from build123d import *

# Parameters (mm, degrees)
BOSS_EXTRUDE1_DEPTH = 11.4
CUT_EXTRUDE1_DEPTH  = 0.6
CHAMFER1_SIZE       = 0.5
CUT_EXTRUDE2_DEPTH  = 6


with BuildPart() as part:
    # Sketch2 → Boss-Extrude1 (new body)
    with BuildSketch(Plane(origin=(0, 0, 0), x_dir=(1, 0, 0), z_dir=(0, 1, 0))):
        with BuildLine():
            Line((-13.742133053, -2.045066795), (-2.112067201, -2.853361551))
            ThreePointArc((-2.112067201, -2.853361551), (0, -3.55), (2.112067201, -2.853361551))
            Line((2.112067201, -2.853361551), (13.742133053, -2.045066795))
            ThreePointArc((13.742133053, -2.045066795), (15.65, 0), (13.742133053, 2.045066795))
            Line((13.742133053, 2.045066795), (2.112067201, 2.853361551))
            ThreePointArc((2.112067201, 2.853361551), (0, 3.55), (-2.112067201, 2.853361551))
            Line((-2.112067201, 2.853361551), (-13.742133053, 2.045066795))
            ThreePointArc((-13.742133053, 2.045066795), (-15.65, 0), (-13.742133053, -2.045066795))
        make_face()
    extrude(amount=BOSS_EXTRUDE1_DEPTH)

    # Sketch3 → Cut-Extrude1 (cut)
    with BuildSketch(Plane.XZ):
        with BuildLine():
            ThreePointArc((-2.112067201, 2.853361551), (0, -3.55), (2.112067201, 2.853361551))
            ThreePointArc((2.112067201, 2.853361551), (0, 3.55), (-2.112067201, 2.853361551))
        make_face()
    extrude(amount=-CUT_EXTRUDE1_DEPTH, mode=Mode.SUBTRACT)

    # Chamfer1
    chamfer1_edges = [part.edges().sort_by_distance(p)[0] for p in [
        (-3.55, 0, 0),
        (3.55, 0, 0),
    ]]
    chamfer(chamfer1_edges, length=CHAMFER1_SIZE)

    # Shaft Key → Cut-Extrude2 (cut)
    with BuildSketch(Plane(origin=(0, 11.4, 0), x_dir=(1, 0, 0), z_dir=(0, 1, 0))):
        with BuildLine():
            Line((1.6, -1.855397532), (1.6, -5.45))
            Line((1.6, -5.45), (-1.6, -5.45))
            Line((-1.6, -5.45), (-1.6, -1.855397532))
            ThreePointArc((-1.6, -1.855397532), (-2.45, 0), (-1.6, 1.855397532))
            Line((-1.6, 1.855397532), (-1.6, 5.45))
            Line((-1.6, 5.45), (1.6, 5.45))
            Line((1.6, 5.45), (1.6, 1.855397532))
            ThreePointArc((1.6, 1.855397532), (2.45, 0), (1.6, -1.855397532))
        make_face()
    extrude(amount=-CUT_EXTRUDE2_DEPTH, mode=Mode.SUBTRACT)


solid = part.part
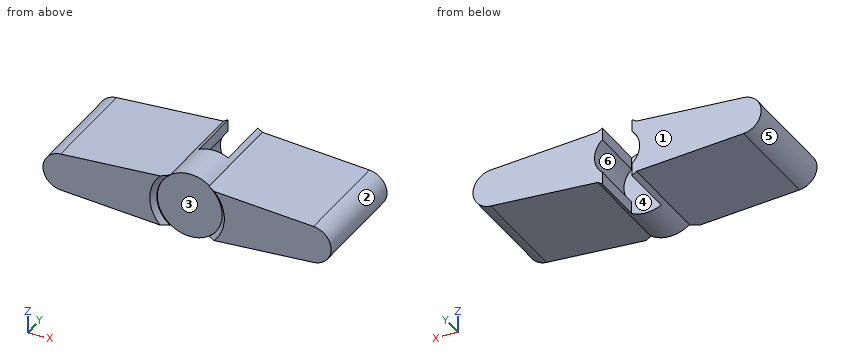
Could you check a few things on this model? Use its own coordinates, in mm. Face numbers are marked on the shaded views. A direction names the side the tool comes from. Give positions to 0.01 mm unless a question says otherwise; leave off trailing zeros. Order: outer loops, then holes, each group sorted by start corner. A loop starts at its lowest first (then second) coordinate and runs counter-clockwise, first axis right, second up.
1. Suppose I cut it at D-D (x = -0.5). Write out the boundary of the cut face in (y, z), plus the area to 3 significant figures.
Answers below:
outline: (0.6, -3.51) - (5.4, -3.51) - (5.4, 3.51) - (0.6, 3.51) - close
area: 33.7 mm2
2. For pin 1 (2.5 mm diameter, centred on x = 0, z = 1, fed in from +Y); pin 2 (1.4 mm diameter, centred on y = 7.5, z = 2.5, fed in from +X); pin 3 (2 mm diameter, centred on x = 1, z = 1.5, fed in from -Y), each with a flat end and sliding along its axis, tell me the tip position at first contact or that it passes through.
Answers below:
pin 1: stops at y = 5.4
pin 2: stops at x = 14.58
pin 3: stops at y = 0.6
3. Suppose I cut it at B-B (y = 3). Write out the boundary of the cut face in (x, z).
Answers below:
outline: (-13.74, -2.05) - (-2.11, -2.85) arc R3.55 ccw to (2.11, -2.85) - (13.74, -2.05) arc R2.05 ccw to (13.74, 2.05) - (2.11, 2.85) arc R3.55 ccw to (-2.11, 2.85) - (-13.74, 2.05) arc R2.05 ccw to start
4. Thinking about a two-plate mould opening in X: for the marked faces 1, 2, 3 and 4, which applies, +X half, -X half, draft (parallel to the pull), parting line (faces both ways), or undercut?
Answers below:
face 1: draft
face 2: +X half
face 3: undercut
face 4: undercut
5. Which directions (+Z, -Z, +X, -X, +Y, -Y) give clear straight access to the entire face, cutting with the end or side of a thin tool? Please do the marked faces 5 and 6.
Answers below:
face 5: -X, +Y, -Y
face 6: +Y
6. Suppose I cut it at C-C (z = 0). Write out the boundary of the cut face in (x, y), plus the area to 3 significant figures.
Answers below:
outline: (-15.65, 0) - (-4.05, 0) - (-3.55, 0.5) - (-3.55, 0.6) - (3.55, 0.6) - (3.55, 0.5) - (4.05, 0) - (15.65, 0) - (15.65, 11.4) - (2.45, 11.4) - (2.45, 5.4) - (-2.45, 5.4) - (-2.45, 11.4) - (-15.65, 11.4) - close
area: 323 mm2
7. I need wall thicknesses on L1, parallel to Y at x = 1.5, z = 1; L2, parallel to X at y = 8.25, z = 0.75; L3, parallel to Z at x = -4, y = 7.25. Which ranges of each line are inside material? Lowest first, please.
Answers below:
L1: y = 0.6 to 5.4
L2: x = -15.51 to -2.33, 2.33 to 15.51
L3: z = -2.72 to 2.72
